Could you check a few things on this model? Use its own coordinates, in mm. Face numbers are marked on the shaded views. A direction names the side the tool comes from. Round coordinates to 2 decimals unless told otherwise and drop trailing zeros. Order: outer loops, then holes, each group sorted by start corner. A loop starts at its lowest first (then second) coordinate and runs counter-clockwise, first axis right, second up. Notation, with made-up numbers: (-9.75, 67.25) - (8.25, 67.25) arc R17 ccw to (8.25, 94.25) - close; hole circle Ø11 at (14, -31.75). An arc over 180 degrees is marked (long way). Use one line per item in the form item = value.
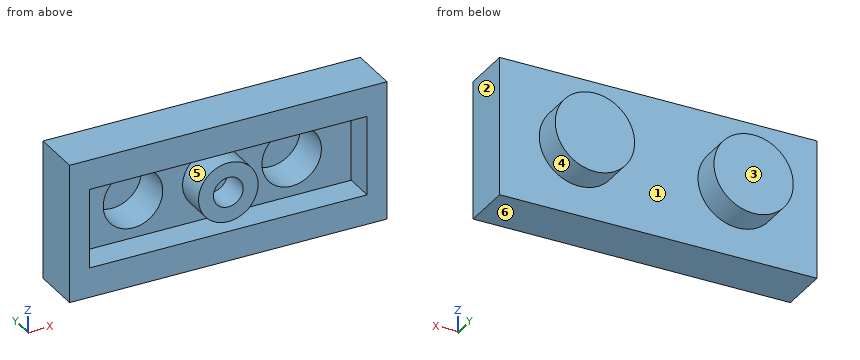
from build123d import *

# Parameters (mm, degrees)
SKETCH1_W           = 20.32
SKETCH1_H           = 3.175
BOSS_EXTRUDE2_DEPTH = 4.445
SKETCH3_R           = 2.54
BOSS_EXTRUDE3_DEPTH = 1.905
SKETCH4_W           = 17.78
SKETCH4_H           = 5.08
CUT_EXTRUDE1_DEPTH  = 1.905
SKETCH5_R           = 1.905
CUT_EXTRUDE2_DEPTH  = 2.54
SKETCH6_R           = 1.905
SKETCH6_R_2         = 0.9525
BOSS_EXTRUDE4_DEPTH = 1.905


with BuildPart() as part:
    # Sketch1 → Boss-Extrude2 (new body, symmetric)
    with BuildSketch(Plane.XY):
        with Locations((0, -1.5875)):
            Rectangle(SKETCH1_W, SKETCH1_H)
    extrude(amount=BOSS_EXTRUDE2_DEPTH, both=True)

    # Sketch3 → Boss-Extrude3 (add)
    with BuildSketch(Plane(origin=(0, 0, 0), x_dir=(1, 0, 0), z_dir=(0, 1, 0))):
        with Locations((-5.08, 0)):
            Circle(SKETCH3_R)
        with Locations((5.08, 0)):
            Circle(SKETCH3_R)
    extrude(amount=BOSS_EXTRUDE3_DEPTH)

    # Sketch4 → Cut-Extrude1 (cut)
    with BuildSketch(Plane.XZ.offset(3.175)):
        Rectangle(SKETCH4_W, SKETCH4_H)
    extrude(amount=-CUT_EXTRUDE1_DEPTH, mode=Mode.SUBTRACT)

    # Sketch5 → Cut-Extrude2 (cut)
    with BuildSketch(Plane.XZ.offset(1.27)):
        with Locations((-5.08, 0)):
            Circle(SKETCH5_R)
        with Locations((5.08, 0)):
            Circle(SKETCH5_R)
    extrude(amount=-CUT_EXTRUDE2_DEPTH, mode=Mode.SUBTRACT)

    # Sketch6 → Boss-Extrude4 (add)
    with BuildSketch(Plane.XZ.offset(1.27)):
        Circle(SKETCH6_R)
        Circle(SKETCH6_R_2, mode=Mode.SUBTRACT)
    extrude(amount=BOSS_EXTRUDE4_DEPTH)


solid = part.part
Item 1: Imagine slicing it at D-D on y = 0.8. Please give me the cut outline in (x, z) (3 decimals), plus the area to 3 significant figures.
Found:
outline = circle Ø5.08 at (-5.08, 0); circle Ø5.08 at (5.08, 0); hole circle Ø3.81 at (-5.08, 0); hole circle Ø3.81 at (5.08, 0)
area = 17.7 mm2
Item 2: Imagine slicing it at A-A on y = -2.35. Please give me the cut outline in (x, z) (1 decimal), plus the area to 3 significant figures.
Found:
outline = (-10.2, -4.4) - (10.2, -4.4) - (10.2, 4.4) - (-10.2, 4.4) - close; circle Ø3.8 at (0, 0); hole (-8.9, -2.5) - (8.9, -2.5) - (8.9, 2.5) - (-8.9, 2.5) - close; hole circle Ø1.9 at (0, 0)
area = 98.9 mm2
Item 3: I need wall thicknesses on L1, parallel to Z at x = -5.5, y = -1.7 (3 decimals); L2, parallel to X at y = 0.45, z = 1.25; L3, parallel to Y at x = 0, z = 4.25 (3 decimals). Which ranges of each line are inside material? Lowest first, please.
Found:
L1 = -4.445 to -2.54, 2.54 to 4.445
L2 = -7.29 to -6.52, -3.64 to -2.87, 2.87 to 3.64, 6.52 to 7.29
L3 = -3.175 to 0
Item 4: Will these pins go through, and if not, where does the flat tip stop? P1, Ø2.5, axis at x = -5.08, z = 0, coming from the -Y side; P2, Ø4, axis at x = -5, z = 0.5, coming from the -Y side; P3, Ø2, axis at x = -0.5, z = 0, coming from the -Y side (3 decimals); P4, Ø1.5, axis at x = 0, z = 0, coming from the +Y side.
Found:
P1 = 1.27
P2 = -1.27
P3 = -3.175
P4 = 0
Item 5: Imagine slicing it at B-B on x = 0. Please give me the cut outline in (y, z) (1 decimal), plus the area to 3 significant figures.
Found:
outline = (-3.2, -4.4) - (0, -4.4) - (0, 4.4) - (-3.2, 4.4) - (-3.2, 2.5) - (-1.3, 2.5) - (-1.3, 1.9) - (-3.2, 1.9) - (-3.2, 1) - (-1.3, 1) - (-1.3, -1) - (-3.2, -1) - (-3.2, -1.9) - (-1.3, -1.9) - (-1.3, -2.5) - (-3.2, -2.5) - close
area = 22.2 mm2
Item 6: If we mould it in two halves opening along X, with no side actions, what happens to the marked faces 1, 2 and 3? For each: released by +X, released by -X, zero draft, split by the parting line, or undercut.
Found:
face_1 = undercut
face_2 = released by +X
face_3 = zero draft
Item 7: For the marked faces 4, 5 and 6, which set-ups out of +Z, -Z, +X, -X, +Y, -Y let a thin tool reach every point of the face, with its end or its side?
Found:
face_4 = +Y
face_5 = -Y
face_6 = -Z, +X, -X, +Y, -Y
